For this review, take the finished solid that the model builds, in its own axes (mm). Face numbers are marked on the shaded views. A direction names the side the tool comes from. Round coordinates to 2 decimals unless told otherwise and drop trailing zeros. Order: outer loops, then holes, each group sorted by start corner. A loop starts at its lowest first (then second) coordinate and runs counter-clockwise, first axis right, second up. Notation, with made-up numbers: M 6,-15 L 52,-15 A14 ccw 52,8 Z; hole C 52,58 d5. An arc over 180 degrees is marked long. Use a Markdown table: item, result.
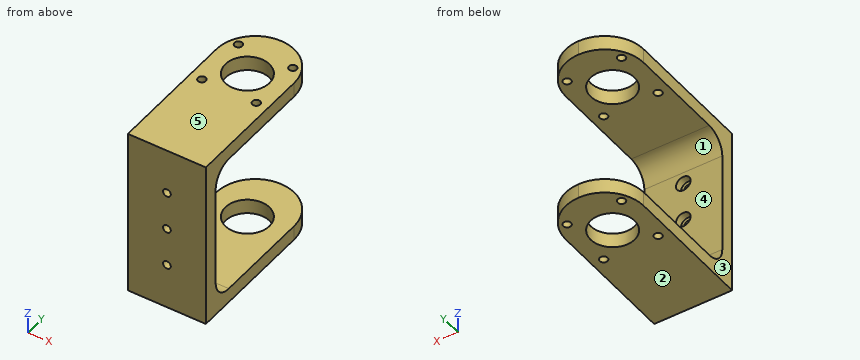
from build123d import *

# Parameters (mm, degrees)
SKETCH1_W           = 50.8
SKETCH1_H           = 110.49
BOSS_EXTRUDE1_DEPTH = 9.525
SKETCH2_W           = 50.8
SKETCH2_H           = 9.525
BOSS_EXTRUDE2_DEPTH = 101.6
SKETCH3_W           = 50.8
SKETCH3_H           = 9.525
BOSS_EXTRUDE3_DEPTH = 101.6
SKETCH8_R           = 14.351
CUT_EXTRUDE7_DEPTH  = 165.734470361
SKETCH9_R           = 2.5527
CUT_EXTRUDE8_DEPTH  = 159.503428512
SKETCH10_R          = 2.5527
CUT_EXTRUDE9_DEPTH  = 6.35
FILLET5_R           = 25.4
FILLET6_R           = 25.4
FILLET7_R           = 25.4
FILLET8_R           = 25.4
SKETCH11_R          = 2.5527
CUT_EXTRUDE10_DEPTH = 159.465264648
SKETCH12_R          = 2.54
CUT_EXTRUDE11_DEPTH = 159.465264648
FILLET9_R           = 12.7
SKETCH13_R          = 4.7625
CUT_EXTRUDE12_DEPTH = 4.826


with BuildPart() as part:
    # Sketch1 → Boss-Extrude1 (new body)
    with BuildSketch(Plane(origin=(0, 0, 0), x_dir=(1, 0, 0), z_dir=(0, 1, 0))):
        with Locations((25.4, 55.245)):
            Rectangle(SKETCH1_W, SKETCH1_H)
    extrude(amount=BOSS_EXTRUDE1_DEPTH)

    # Sketch2 → Boss-Extrude2 (add)
    with BuildSketch(Plane(origin=(0, 9.525, 0), x_dir=(1, 0, 0), z_dir=(0, 1, 0))):
        with Locations((25.4, 105.7275)):
            Rectangle(SKETCH2_W, SKETCH2_H)
    extrude(amount=BOSS_EXTRUDE2_DEPTH)

    # Sketch3 → Boss-Extrude3 (add)
    with BuildSketch(Plane(origin=(0, 9.525, 0), x_dir=(1, 0, 0), z_dir=(0, 1, 0))):
        with Locations((25.4, 4.7625)):
            Rectangle(SKETCH3_W, SKETCH3_H)
    extrude(amount=BOSS_EXTRUDE3_DEPTH)

    # Sketch8 → Cut-Extrude7 (cut, through all)
    with BuildSketch(Plane.XY):
        with Locations((25.4, 78.105)):
            Circle(SKETCH8_R)
    extrude(amount=-CUT_EXTRUDE7_DEPTH, mode=Mode.SUBTRACT)

    # Sketch9 → Cut-Extrude8 (cut, through all)
    with BuildSketch(Plane(origin=(0, 0, -9.525), x_dir=(-1, 0, 0), z_dir=(0, 0, -1))):
        with Locations((-43.1292, 95.8342)):
            Circle(SKETCH9_R)
        with Locations((-7.6708, 95.8342)):
            Circle(SKETCH9_R)
        with Locations((-7.6708, 60.3758)):
            Circle(SKETCH9_R)
        with Locations((-43.1292, 60.3758)):
            Circle(SKETCH9_R)
    extrude(amount=-CUT_EXTRUDE8_DEPTH, mode=Mode.SUBTRACT)

    # Sketch10 → Cut-Extrude9 (cut)
    with BuildSketch(Plane(origin=(0, 0, -110.49), x_dir=(-1, 0, 0), z_dir=(0, 0, -1))):
        with Locations((-43.1292, 95.8342)):
            Circle(SKETCH10_R)
        with Locations((-7.6708, 95.8342)):
            Circle(SKETCH10_R)
        with Locations((-7.6708, 60.3758)):
            Circle(SKETCH10_R)
        with Locations((-43.1292, 60.3758)):
            Circle(SKETCH10_R)
    extrude(amount=-CUT_EXTRUDE9_DEPTH, mode=Mode.SUBTRACT)

    # Fillet5
    fillet5_edges = [part.edges().sort_by_distance(p)[0] for p in [
        (0, 111.125, -4.7625),
    ]]
    fillet(fillet5_edges, radius=FILLET5_R)

    # Fillet6
    fillet6_edges = [part.edges().sort_by_distance(p)[0] for p in [
        (50.8, 111.125, -4.7625),
    ]]
    fillet(fillet6_edges, radius=FILLET6_R - 0.0001)  # a hair under: the kernel refuses the full size

    # Fillet7
    fillet7_edges = [part.edges().sort_by_distance(p)[0] for p in [
        (0, 111.125, -105.7275),
    ]]
    fillet(fillet7_edges, radius=FILLET7_R)

    # Fillet8
    fillet8_edges = [part.edges().sort_by_distance(p)[0] for p in [
        (50.8, 111.125, -105.7275),
    ]]
    fillet(fillet8_edges, radius=FILLET8_R - 0.0001)  # a hair under: the kernel refuses the full size

    # Sketch11 → Cut-Extrude10 (cut, through all)
    with BuildSketch(Plane(origin=(0, 9.525, 0), x_dir=(1, 0, 0), z_dir=(0, 1, 0))):
        with Locations(Location((25.4, 55.245, 0), (0, 0, 270))):
            Circle(SKETCH11_R)
    extrude(amount=-CUT_EXTRUDE10_DEPTH, mode=Mode.SUBTRACT)

    # Sketch12 → Cut-Extrude11 (cut, through all)
    with BuildSketch(Plane(origin=(0, 9.525, 0), x_dir=(1, 0, 0), z_dir=(0, 1, 0))):
        with Locations(Location((25.4, 29.845, 0), (0, 0, 270))):
            Circle(SKETCH12_R)
        with Locations(Location((25.4, 80.645, 0), (0, 0, 270))):
            Circle(SKETCH12_R)
    extrude(amount=-CUT_EXTRUDE11_DEPTH, mode=Mode.SUBTRACT)

    # Fillet9
    fillet9_edges = [part.edges().sort_by_distance(p)[0] for p in [
        (25.4, 9.525, -100.965),
        (25.4, 9.525, -9.525),
    ]]
    fillet(fillet9_edges, radius=FILLET9_R)

    # Sketch13 → Cut-Extrude12 (cut)
    with BuildSketch(Plane(origin=(0, 9.525, 0), x_dir=(1, 0, 0), z_dir=(0, 1, 0))):
        with Locations(Location((25.4, 55.245, 0), (0, 0, 270))):
            Circle(SKETCH13_R)
        with Locations(Location((25.4, 29.845, 0), (0, 0, 270))):
            Circle(SKETCH13_R)
        with Locations(Location((25.4, 80.645, 0), (0, 0, 270))):
            Circle(SKETCH13_R)
    extrude(amount=-CUT_EXTRUDE12_DEPTH, mode=Mode.SUBTRACT)


solid = part.part
Q1. Machinability: for the marked faces 4 and 5, which of the approach directions +Z, -Z, +X, -X, +Y, -Y give a long, thin tool a straight path to every point of the face, cutting with its end or side? Answer none if there is none.
Determined:
| item | result |
|---|---|
| face 4 | +X, -X, +Y |
| face 5 | +Z, +X, -X, +Y, -Y |
Q2. Add section D-D (x = 13). Write out the cut boundary in (y, z) (3 decimals), then the cut area to 3 significant figures.
Determined:
| item | result |
|---|---|
| outline | M 0,-110.49 L 70.881,-110.49 L 70.881,-100.965 L 22.225,-100.965 A12.7 cw 9.525,-88.265 L 9.525,-22.225 A12.7 cw 22.225,-9.525 L 70.881,-9.525 L 70.881,0 L 0,0 Z; M 85.329,-110.49 L 107.893,-110.49 L 107.893,-100.965 L 85.329,-100.965 Z; M 85.329,-9.525 L 107.893,-9.525 L 107.893,0 L 85.329,0 Z |
| area | 2,720 mm^2 |
Q3. Clearance check with flat-ended pins moving along their axes: pin 1 (7.5 mm diameter, centred on x = 25, z = -82.5, fed in from +Y) (3 decimals); pin 2 (5 mm diameter, centred on x = 26, z = -54, fed in from +Y); pin 3 (2.5 mm diameter, centred on x = 42.5, y = 96.5, fed in from -Z). State where each tip first meets the part, or that it passes through.
Determined:
| item | result |
|---|---|
| pin 1 | stops at y = 9.525 |
| pin 2 | stops at y = 4.7 |
| pin 3 | stops at z = -104.14 |
Q4. Add section A-A (y = 54). Write out the cut boundary in (x, z) (3 decimals), then the cut area to 3 significant figures.
Determined:
| item | result |
|---|---|
| outline | M 0,-110.49 L 50.8,-110.49 L 50.8,-100.965 L 0,-100.965 Z; M 0,-9.525 L 50.8,-9.525 L 50.8,0 L 0,0 Z |
| area | 968 mm^2 |
Q5. Add section C-C (z = -8). Give the number of separate pieces and of enclosed holes in the cut face, then the cut area to 3 significant figures.
Determined:
| item | result |
|---|---|
| separate pieces | 1 |
| enclosed holes | 5 |
| area | 4,640 mm^2 |
Q6. Draft analysis for pull direction Z (two halves, no side actions). For the marked faces 1, 2 and 3, state which applies: pulls with the +Z half, pulls with the -Z half, needs draft (parallel to the pull), parting line crosses it, or undercut.
Determined:
| item | result |
|---|---|
| face 1 | undercut |
| face 2 | pulls with the -Z half |
| face 3 | needs draft |
Q7. Add section B-B (x = 36). Write out the cut boundary in (y, z) (1 decimal), then the cut area to 3 significant figures.
Determined:
| item | result |
|---|---|
| outline | M 0,-110.5 L 68.4,-110.5 L 68.4,-101 L 22.2,-101 A12.7 cw 9.5,-88.3 L 9.5,-22.2 A12.7 cw 22.2,-9.5 L 68.4,-9.5 L 68.4,0 L 0,0 Z; M 87.8,-110.5 L 108.8,-110.5 L 108.8,-101 L 87.8,-101 Z; M 87.8,-9.5 L 108.8,-9.5 L 108.8,0 L 87.8,0 Z |
| area | 2,640 mm^2 |
Q8. Wall thickness on line 1 along Y through (x, z) = (8, -5); line 2 along Z through (x, y) = (3, 55) (3 decimals); line 3 along Z through (x, y) = (21, 5): over which ranges is each line inside the solid? List them lowest first. Write a range as [from, to].
Determined:
| item | result |
|---|---|
| line 1 | y = [0, 57.84], [62.91, 93.3], [98.37, 104.23] |
| line 2 | z = [-110.49, -100.965], [-9.525, 0] |
| line 3 | z = [-110.49, -82.47], [-78.82, -57.07], [-53.42, -31.67], [-28.02, 0] |
